from build123d import *

# Parameters (mm, degrees)
PAD002_DEPTH    = 10
FILLET010_R     = 3
FILLET011_R     = 3
FILLET012_R     = 1
SKETCH002_R     = 1.25
POCKET001_DEPTH = 2.001


with BuildPart() as part:
    # CopyCopySketch004 → Pad002 (new body)
    with BuildSketch(Plane.YZ):
        Polygon((-6, 3), (-6, 13), (6, 13), (6, 3), (18, 3), (18, 5), (8, 5), (8, 15), (-8, 15), (-8, 5), (-18, 5), (-18, 3), align=None)
    extrude(amount=PAD002_DEPTH)

    # Fillet010
    fillet010_edges = [part.edges().sort_by_distance(p)[0] for p in [
        (5, -6, 13),
    ]]
    fillet(fillet010_edges, radius=FILLET010_R)

    # Fillet011
    fillet011_edges = [part.edges().sort_by_distance(p)[0] for p in [
        (5, 6, 13),
    ]]
    fillet(fillet011_edges, radius=FILLET011_R)

    # Fillet012
    fillet012_edges = [part.edges().sort_by_distance(p)[0] for p in [
        (5, 18, 5),
        (5, 8, 15),
        (5, -8, 15),
        (5, -18, 5),
    ]]
    fillet(fillet012_edges, radius=FILLET012_R)

    # Sketch002 (on Face17 of Fillet012) → Pocket001 (cut, through all)
    with BuildSketch(Plane(origin=(0, 0, 5), x_dir=(0, -1, 0), z_dir=(0, 0, 1))):
        with Locations((14, 5)):
            Circle(SKETCH002_R)
        with Locations((-14, 5)):
            Circle(SKETCH002_R)
    extrude(amount=-POCKET001_DEPTH, mode=Mode.SUBTRACT)


with BuildPart() as part_1:
    # Body003 placement: moved
    add(part.part.moved(Location((-54.676946, -34.731148, 0))))


solid = part_1.part
Verification items for the finished model (mm, model axes). A direction names the side the tool comes from. Coordinates: 2 decimals unless noted, no trailing zeros. Write each loop counter-clockwise with the first axis right and the second up, starting at its lowest first coordinate (ties: lowest second). Pieces come first, ordered by that corner, then holes. Notation, with made-up numbers: M -18.75,42.25 L 1.25,42.25 A19 cw 1.25,63.25 Z; hole C -10.5,61 d9. An arc over 180 degrees is marked long. One line per question, with ' | ' between items.
1) Material ranges on L1, parallel to Y at x = -51, z = 5.25; L2, parallel to Y at x = -53, z = 3.5; L3, parallel to Z at x = -48.75, y = -22.5, recorded low to high.
Solutions:
L1: -42.73 to -40.73, -28.73 to -26.73 | L2: -52.73 to -40.73, -28.73 to -16.73 | L3: 3 to 5
2) Release check for a two-part mould opening along X. For faces 1 (the face through (-48.438, -20.568, 4.014)), 2 (the face through (-48.83, -47.81, 4.01)), 3 (the face through (-50, -47, 3)), 4 (the face through (-44.677, -34.8, 13.5)) record: +X half, -X half, draft (parallel to the pull), parting line (faces both ways), or undercut.
Solutions:
face 1: undercut | face 2: undercut | face 3: draft | face 4: +X half
3) Depth check by flat-ended pin: pin 1 Ø1.5 at (x, y) = (-49.68, -20.73) entering from -Z; pin 2 Ø2.5 at (x, y) = (-48.5, -22) entering from +Z; pin 3 Ø3 at (x, y) = (-49.68, -48.73) entering from -Z; pin 4 Ø5 at (x, z) = (-51, 11) entering from +Y. Enter the tip coordinate at first touch or a pass-through.
Solutions:
pin 1: through | pin 2: z = 5 | pin 3: z = 3 | pin 4: y = -26.73
4) Sectioned sample at A-A on z = 7.25. Record the cut outline in (x, y), then the cut area to 3 significant figures.
Solutions:
outline: M -54.68,-42.73 L -44.68,-42.73 L -44.68,-40.73 L -54.68,-40.73 Z; M -54.68,-28.73 L -44.68,-28.73 L -44.68,-26.73 L -54.68,-26.73 Z | area: 40.0 mm^2
5) Sectioned sample at C-C on x = -48.75. Record the cut outline in (y, z).
Solutions:
outline: M -52.73,3 L -49.57,3 L -49.57,5 L -51.73,5 A1 ccw -52.73,4 Z; M -47.89,3 L -40.73,3 L -40.73,10 A3 cw -37.73,13 L -31.73,13 A3 cw -28.73,10 L -28.73,3 L -21.57,3 L -21.57,5 L -26.73,5 L -26.73,14 A1 ccw -27.73,15 L -41.73,15 A1 ccw -42.73,14 L -42.73,5 L -47.89,5 Z; M -19.89,3 L -16.73,3 L -16.73,4 A1 ccw -17.73,5 L -19.89,5 Z
6) Access from +Z, -Z, +X, -X, +Y, -Y to the whole of each face (thin tool, end or side, straight path). Record for faces 5 (the face through (-50, -47, 5)), 6 (the face through (-50, -23, 3)), 7 (the face through (-50, -40.731, 6)), 8 (the face through (-50, -26.731, 9)).
Solutions:
face 5: +Z, +X, -X, -Y | face 6: -Z, +X, -X, +Y, -Y | face 7: -Z, +X, -X | face 8: +Z, +X, -X, +Y
7) Sectioned sample at B-B on x = -46.5. Record the cut outline in (y, z), then the cut area to 3 significant figures.
Solutions:
outline: M -52.73,3 L -40.73,3 L -40.73,10 A3 cw -37.73,13 L -31.73,13 A3 cw -28.73,10 L -28.73,3 L -16.73,3 L -16.73,4 A1 ccw -17.73,5 L -26.73,5 L -26.73,14 A1 ccw -27.73,15 L -41.73,15 A1 ccw -42.73,14 L -42.73,5 L -51.73,5 A1 ccw -52.73,4 Z | area: 115 mm^2
8) Sectioned sample at D-D on z = 12.5. Record the cut outline in (x, y), then the cut area to 3 significant figures.
Solutions:
outline: M -54.68,-42.73 L -44.68,-42.73 L -44.68,-39.39 L -54.68,-39.39 Z; M -54.68,-30.07 L -44.68,-30.07 L -44.68,-26.73 L -54.68,-26.73 Z | area: 66.8 mm^2
